```python
from build123d import *

# Parameters (mm, degrees)
F0_R     = 20
F0_R_2   = 10
F4_R     = 30
F4_R_2   = 20
F5_DEPTH = 3
F7_R     = 30
F7_R_2   = 20
F8_DEPTH = 10


with BuildPart() as f2:
    # F2: sweep along a path in F1
    with BuildLine(Plane.XZ) as f2_path:
        Line((0, 0), (20, 0))
        ThreePointArc((20, 0), (48.2842712475, -11.7157287525), (60, -40))
        Line((60, -40), (60, -65.3837376879))
    # F0 (on Right) → F2 (sweep)
    with BuildSketch(Plane.YZ):
        Circle(F0_R)
        Circle(F0_R_2, mode=Mode.SUBTRACT)
    sweep(path=f2_path.line)

    # F4 (on offset) → F5 (join)
    with BuildSketch(Plane(origin=(3, 0, 0), x_dir=(0, -1, 0), z_dir=(-1, 0, 0))):
        Circle(F4_R)
        Circle(F4_R_2, mode=Mode.SUBTRACT)
    extrude(amount=-F5_DEPTH)

    # F7 (on offset) → F8 (join)
    with BuildSketch(Plane(origin=(0, 0, -62.3837376879), x_dir=(1, 0, 0), z_dir=(0, 0, -1))):
        with Locations((60, 0)):
            Circle(F7_R)
        with Locations((60, 0)):
            Circle(F7_R_2, mode=Mode.SUBTRACT)
    extrude(amount=-F8_DEPTH)


solid = f2.part
```
Input: part model. Units: mm. Frame: model coordinates. A direction names the side the tool comes from. Coordinates: 2 decimals unless noted, no trailing zeros. Order: outer loops, then holes, each group sorted by start corner. A loop starts at its lowest first (then second) coordinate and runs counter-clockwise, first axis right, second up. Notation, with made-up numbers: (43.25, 2) - (63.25, 2) arc R14 ccw to (63.25, 26) - close; hole circle Ø11 at (48, 80). An arc over 180 degrees is marked (long way). Return JSON: item names as keys, results as strings.
Q1. Cut plane A-A (y = -24). Return loops of the section in (x, z).
The answers:
{"outline": "(3, -18) - (6, -18) - (6, 18) - (3, 18) - close; (42, -62.38) - (78, -62.38) - (78, -52.38) - (42, -52.38) - close"}
Q2. Draft query along X for faces 4 (the flat face through (69, 5, -65.384)), 5 (the flat face through (6, -6, -20)), 6 (the cylindrical face through (42.257, 9.229, -46.279)). Return one class per face: +X half, -X half, draft (parallel to the pull), parting line (faces both ways), or undercut.
The answers:
{"face 4": "draft", "face 5": "undercut", "face 6": "parting line"}
Q3. Cut plane C-C (y = 12.5). Return loops of the section in (x, z).
The answers:
{"outline": "(0, -15.61) - (3, -15.61) - (3, -27.27) - (6, -27.27) - (6, -15.61) - (20, -15.61) arc R24.39 cw to (44.39, -40) - (44.39, -52.38) - (32.73, -52.38) - (32.73, -62.38) - (44.39, -62.38) - (44.39, -65.38) - (75.61, -65.38) - (75.61, -62.38) - (87.27, -62.38) - (87.27, -52.38) - (75.61, -52.38) - (75.61, -40) arc R55.61 ccw to (20, 15.61) - (6, 15.61) - (6, 27.27) - (3, 27.27) - (3, 15.61) - (0, 15.61) - close"}
Q4. Ray query, probe 1 along Y at (x, z) = (60, -52); probe 2 along Y at (x, z) = (60, -57); probe 3 along X at (y, z) = (24.5, -16). Return the intervals inside material, ascending.
The answers:
{"probe 1": "y = -20 to -10, 10 to 20", "probe 2": "y = -30 to -10, 10 to 30", "probe 3": "x = 3 to 6"}
Q5. Cut plane D-D (x = 81.5). Return loops of the section in (y, z).
The answers:
{"outline": "(-20.92, -62.38) - (20.92, -62.38) - (20.92, -52.38) - (-20.92, -52.38) - close"}
Q6. First-contact query: pin 1 (12 mm diameter, centred on x = 60, y = 0, fed in from +Z); pin 2 (5 mm diameter, centred on x = 40, y = -8.5, fed in from +Z); pin 3 (10 mm diameter, centred on y = -13.5, z = -45.5, fed in from +X). Flat tips, straight axial feed; report the tip coordinate or a pass-through.
The answers:
{"pin 1": "stops at z = 9.44", "pin 2": "stops at z = 15.94", "pin 3": "stops at x = 78.1"}
Q7. Access query for faces 1 (the cylindrical face through (10.14, -2.17, -9.76)), 2 (the cylindrical face through (30.03, -1.32, -57.45)), 3 (the flat face through (66, 20, -52.384)). Directions: +Z, -Z, +X, -X, +Y, -Y. A direction counts if a zero-diameter tool reaches every point of the face in a straight line with its end or side. Return the directions, or none.
The answers:
{"face 1": "-X", "face 2": "-Z", "face 3": "none"}
